The drawing under review shows one solid part. Ordinate dimensions are in mm from its lowest x, y, z. A direction names the side the tool comes from. Coordinates: 2 decimals unless noted, no trailing zeros. Write each loop counter-clockwise with the first axis right and the second up, starting at its lowest first coordinate (ties: lowest second). Pieces come first, ordered by that corner, then holes.
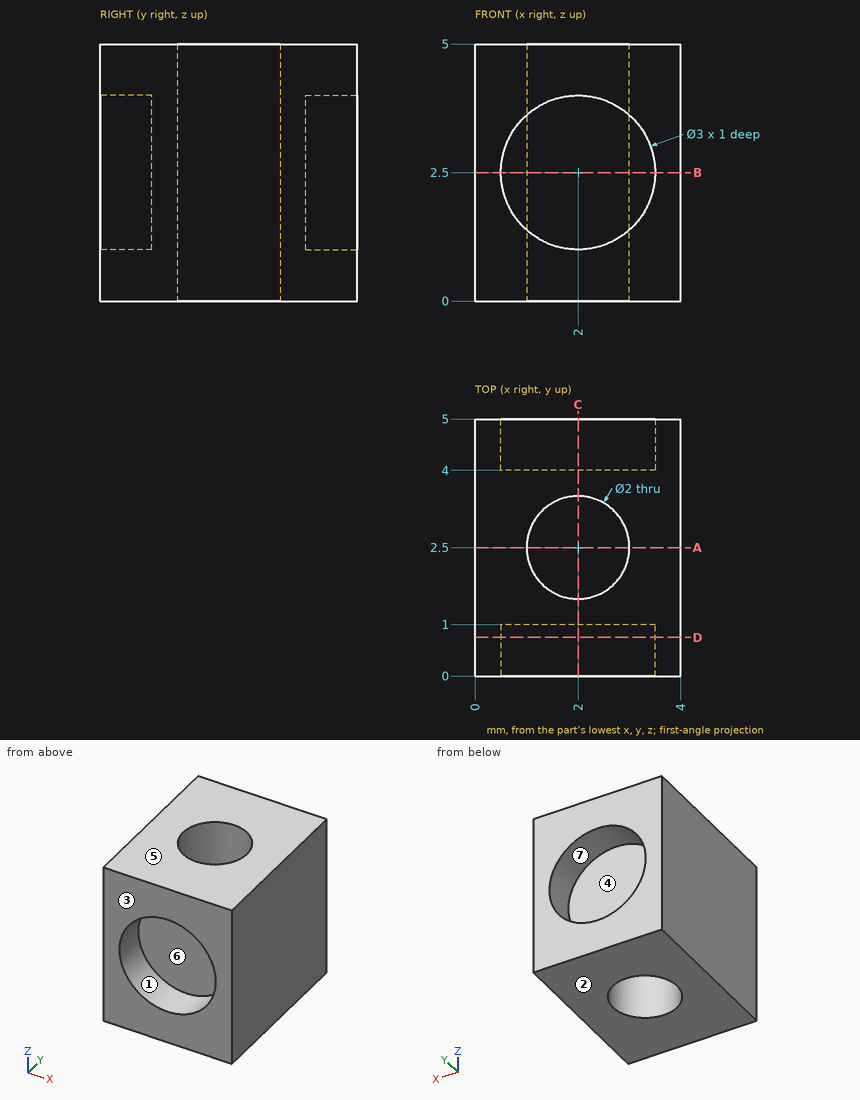
1) For L1, parallel to Z at x = 2, y = 4.25; L2, parallel to Y at x = 1.95, z = 0.85; L3, parallel to X at y = 0.5, z = 2.5, list the stretches that pass through material, from the lowest coordinate up.
2) Tool access review of the marked faces 5, 6 and 7: name each direction out of +Z, -Z, +X, -X, +Y, -Y from which nothing blocks a thin tool from reaching the whole face with its end or side.
3) Consider section B-B (z = 2.5). Give the boundary of the cut face in (x, y), then the cut area to 3 significant figures.
4) The part is to be moulded in two halves that separate along Z. For the marked faces 1, 2, 3 and 4, say which applies: pulls with the +Z half, pulls with the -Z half, needs draft (parallel to the pull), parting line crosses it, or undercut.
5) Consider section C-C (x = 2). Give the boundary of the cut face in (y, z).
6) Clearance check with flat-ended pins moving along their axes: P1, Ø1.8, axis at x = 2, y = 2.5, coming from the +Z side; P2, Ø0.9, axis at x = 2, z = 3, coming from the -Y side. State where each tip first meets the part, or that it passes through.
7) Consider section D-D (y = 0.75). Give the boundary of the cut face in (x, z).
8) Consider section A-A (y = 2.5). Give the boundary of the cut face in (x, z), then the cut area to 3 significant figures.
Results:
1. L1: z = 0 to 1, 4 to 5
1. L2: y = 0 to 1.5, 3.5 to 5
1. L3: x = 0 to 0.5, 3.5 to 4
2. face 5: +Z, +X, -X, +Y, -Y
2. face 6: -Y
2. face 7: +Y
3. outline: (0, 0) - (0.5, 0) - (0.5, 1) - (3.5, 1) - (3.5, 0) - (4, 0) - (4, 5) - (3.5, 5) - (3.5, 4) - (0.5, 4) - (0.5, 5) - (0, 5) - close; hole circle Ø2 at (2, 2.5)
3. area: 10.9 mm2
4. face 1: undercut
4. face 2: pulls with the -Z half
4. face 3: needs draft
4. face 4: undercut
5. outline: (0, 0) - (1.5, 0) - (1.5, 5) - (0, 5) - (0, 4) - (1, 4) - (1, 1) - (0, 1) - close; (3.5, 0) - (5, 0) - (5, 1) - (4, 1) - (4, 4) - (5, 4) - (5, 5) - (3.5, 5) - close
6. P1: passes through
6. P2: stops at y = 1
7. outline: (0, 0) - (4, 0) - (4, 5) - (0, 5) - close; hole circle Ø3 at (2, 2.5)
8. outline: (0, 0) - (1, 0) - (1, 5) - (0, 5) - close; (3, 0) - (4, 0) - (4, 5) - (3, 5) - close
8. area: 10.0 mm2
